```python
from build123d import *

# Parameters (mm, degrees)
SKIZZE1_W                                            = 90
SKIZZE1_H                                            = 90
AUFSATZ_LINEAR_AUSTRAGEN1_DEPTH                      = 1
AUFSATZ_LINEAR_START                                 = -1
SKIZZE12_R                                           = 5
AUFSATZ_LINEAR_AUSTRAGEN2_DEPTH                      = 16
SKIZZE13_R                                           = 2.5
SCHNITT_LINEAR_AUSTRAGEN6_DEPTH                      = 100
LINEARES_MUSTER1_COUNT                               = 2
LINEARES_MUSTER1_PITCH                               = 85
LINEARES_MUSTER1_COUNT_DIR2                          = 2
LINEARES_MUSTER1_PITCH_DIR2                          = 85
AUFSATZ_LINEAR_AUSTRAGEN3_DEPTH                      = 5
AUFSATZ_LINEAR_AUSTRAGEN3_DEPTH_BACK                 = 1
SKIZZE16_R                                           = 4.5
FORMSENKUNG_F_R_M3_LINSENSENKSCHRAUBE_MI_D           = 3.3
FORMSENKUNG_F_R_M3_LINSENSENKSCHRAUBE_MI_DEPTH       = 20
FORMSENKUNG_F_R_M3_LINSENSENKSCHRAUBE_MI_CSINK_D     = 4.2
FORMSENKUNG_F_R_M3_LINSENSENKSCHRAUBE_MI_CSINK_ANGLE = 90
FORMSENKUNG_F_R_M3_LINSENSENKSCHRAUBE_MI_TIP         = 0.991420021


with BuildPart() as part:
    # Skizze1 → Aufsatz-Linear austragen1 (new body)
    with BuildSketch(Plane.XY):
        Rectangle(SKIZZE1_W, SKIZZE1_H)
    extrude(amount=AUFSATZ_LINEAR_AUSTRAGEN1_DEPTH)

    # Skizze12 → Aufsatz-Linear austragen2 (add)
    with BuildSketch(Plane.XY.offset(1).offset(AUFSATZ_LINEAR_START)):
        with Locations((-42.5, 42.5)):
            Circle(SKIZZE12_R)
    aufsatz_linear_austragen2 = extrude(amount=AUFSATZ_LINEAR_AUSTRAGEN2_DEPTH)

    # Skizze13 → Schnitt-Linear austragen6 (cut)
    with BuildSketch(Plane.XY.offset(16)):
        with Locations((-42.5, 42.5)):
            Circle(SKIZZE13_R)
    schnitt_linear_austragen6 = extrude(amount=-SCHNITT_LINEAR_AUSTRAGEN6_DEPTH, mode=Mode.SUBTRACT)

    # Lineares Muster1: Aufsatz-Linear austragen2, Schnitt-Linear austragen6 2 × 2
    with Locations(*[(i * LINEARES_MUSTER1_PITCH, -j * LINEARES_MUSTER1_PITCH_DIR2, 0) for i in range(LINEARES_MUSTER1_COUNT) for j in range(LINEARES_MUSTER1_COUNT_DIR2) if (i, j) != (0, 0)]):
        add(aufsatz_linear_austragen2)
        add(schnitt_linear_austragen6, mode=Mode.SUBTRACT)

    # Skizze16 → Aufsatz-Linear austragen3 (add, two sides: drawn at the far end of the back side and taken through both)
    with BuildSketch(Plane.XY.offset(1).offset(-AUFSATZ_LINEAR_AUSTRAGEN3_DEPTH_BACK)):
        with Locations((44.194173824, -5.303300859)):
            Circle(SKIZZE16_R)
        with Locations((5.303300859, -44.194173824)):
            Circle(SKIZZE16_R)
        with Locations((-44.194173824, 5.303300859)):
            Circle(SKIZZE16_R)
        with Locations((-5.303300859, 44.194173824)):
            Circle(SKIZZE16_R)
    extrude(amount=AUFSATZ_LINEAR_AUSTRAGEN3_DEPTH + AUFSATZ_LINEAR_AUSTRAGEN3_DEPTH_BACK)

    # Formsenkung für M3 Linsensenkschraube mit Schlitz1
    with Locations(Plane.XY.offset(6)):
        with Locations((5.243612969, -44.154400898), (44.194173824, -5.303300859), (-5.303300859, 44.194173824), (-44.194173824, 5.303300859)):
            CounterSinkHole(FORMSENKUNG_F_R_M3_LINSENSENKSCHRAUBE_MI_D / 2, FORMSENKUNG_F_R_M3_LINSENSENKSCHRAUBE_MI_CSINK_D / 2, depth=FORMSENKUNG_F_R_M3_LINSENSENKSCHRAUBE_MI_DEPTH, counter_sink_angle=FORMSENKUNG_F_R_M3_LINSENSENKSCHRAUBE_MI_CSINK_ANGLE)
            with Locations((0, 0, -(FORMSENKUNG_F_R_M3_LINSENSENKSCHRAUBE_MI_DEPTH + FORMSENKUNG_F_R_M3_LINSENSENKSCHRAUBE_MI_TIP / 2))):  # 118° drill point
                Cone(0, FORMSENKUNG_F_R_M3_LINSENSENKSCHRAUBE_MI_D / 2, FORMSENKUNG_F_R_M3_LINSENSENKSCHRAUBE_MI_TIP, mode=Mode.SUBTRACT)


solid = part.part
```
The listing builds one solid part. Answer for the finished solid, in the listing's coordinates (mm). A direction names the side the tool comes from. Coordinates: 2 decimals unless noted, no trailing zeros. Loops run counter-clockwise (first coordinate to the right, second up) from the corner with the lowest first, then second, coordinate; pieces in that order, holes last. Notation, with made-up numbers: M 18,87 L 30,87 A24 cw 30,111 Z; hole C 48,-38.75 d7. An arc over 180 degrees is marked long. Answer as CSV lines item,"result". Start each with the question number.
(1) The part is cut by section B-B (z = 4). State how many separate pieces and enclosed holes the cut face has, and give its area (3 significant figures).
(2) The part is cut by section A-A (z = 10.75). Give the vertices of the cut face in (x, y).
(3) Find the intervals of material crossed by L1, parallel to Y at x = 42.5, z = 8; L2, parallel to Y at x = -44.5, z = 1.75; L3, parallel to Z at x = 25, y = -31, in increasing order. Write a range as [from, to].
(4) Given pin 1 (10 mm diameter, centred on x = -45.5, y = 3.5, fed in from +Z); pin 2 (6 mm diameter, centred on x = 36.5, z = 10.5, fed in from -Y); pin 3 (0.5 mm diameter, centred on x = 31, z = 0.5, fed in from -Y); pin 4 (2.5 mm diameter, centred on x = 5.24, y = -44.15, fed in from -Z), each flat-ended and moving along its own axis, determine where each tip first touches the part or whether it passes through.
(5) The part is cut by section C-C (y = -30). Give the vertices of the cut face in (x, z), and give its area (3 significant figures).
(6) The mould has two halves that part along X. Classify faces 1 (the cylindrical face through (44.81, -43.46, 8.11)), 2 (the flat face through (-45, -44, 16)), 3 (the cylindrical face through (-47.77, 2.57, 2.96)): pulls with the +X half, pulls with the -X half, needs draft (parallel to the pull), parting line crosses it, or undercut.
(7) For faces 4 (the cylindrical face through (4.328, -48.587, 2.958)), 5 (the flat face through (-42, 4, 6)), 6 (the flat face through (-1, 1, 0)), 7 (the flat face through (-4, 42, 6)), determine the directions among +Z, -Z, +X, -X, +Y, -Y from which every point of the face is accessible in a straight line to the end or side of a thin tool.
Determined:
1,separate pieces,"8"
1,enclosed holes,"8"
1,area,"456 mm2"
2,outline,"C -42.5,-42.5 d10; C -42.5,42.5 d10; C 42.5,-42.5 d10; C 42.5,42.5 d10; hole C -42.5,-42.5 d5; hole C -42.5,42.5 d5; hole C 42.5,-42.5 d5; hole C 42.5,42.5 d5"
3,L1,"[-47.5, -45], [-40, -37.5], [37.5, 40], [45, 47.5]"
3,L2,"[-47.08, -44], [-41, -37.92], [0.81, 3.68], [6.92, 9.79], [37.92, 41], [44, 47.08]"
3,L3,"[0, 1]"
4,pin 1,"z = 6"
4,pin 2,"y = -46.5"
4,pin 3,"y = -45"
4,pin 4,"through"
5,outline,"M -45,0 L 45,0 L 45,1 L -45,1 Z"
5,area,"90.0 mm2"
6,face 1,"undercut"
6,face 2,"needs draft"
6,face 3,"parting line crosses it"
7,face 4,"+Z"
7,face 5,"+Z, +X, -X"
7,face 6,"-Z, +X, -X, +Y, -Y"
7,face 7,"+Z, +Y, -Y"
